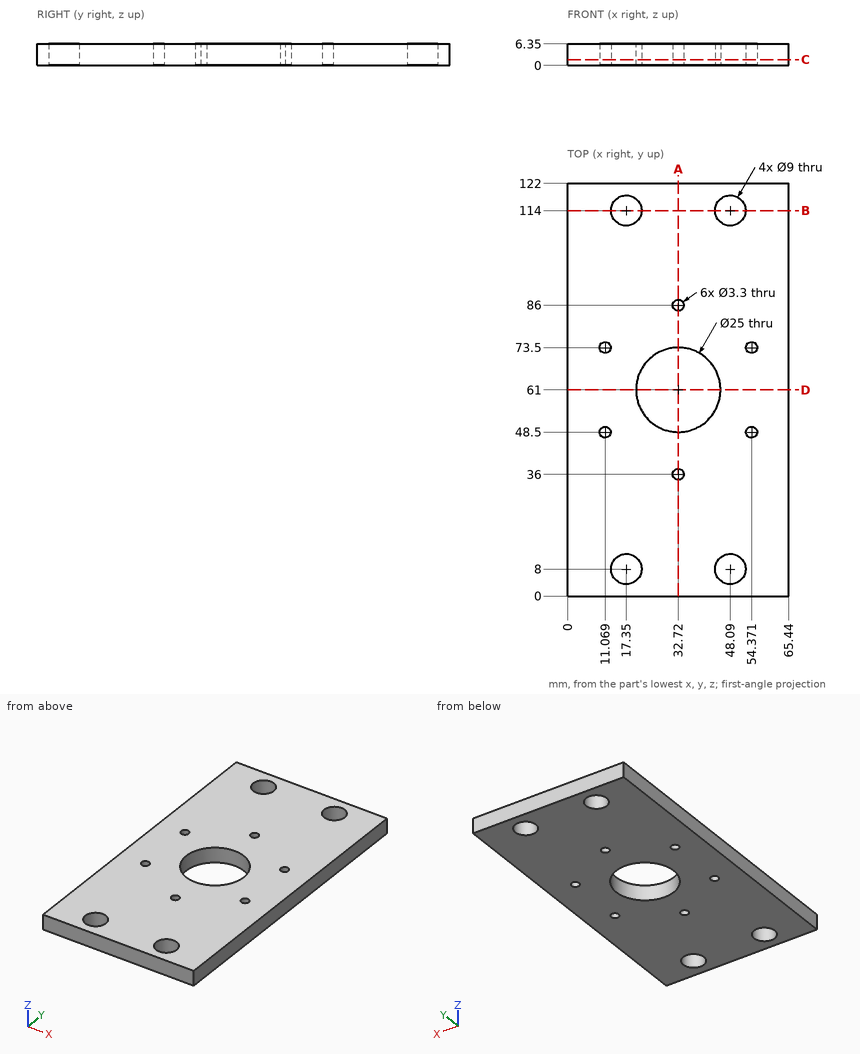
Study the drawing (mm; zero at the part's minimum x, y, z) and answer. Coordinates: 2 decimals unless noted, no trailing zeros. Write each loop counter-clockwise with the first axis right and the second up, starting at its lowest first coordinate (ties: lowest second). Pieces come first, ordered by that corner, then holes.
Q1. Section D-D, the plane y = 61 is taken. Write down the section's boundary in (x, z).
Returned:
outline: (0, 0) - (20.22, 0) - (20.22, 6.35) - (0, 6.35) - close; (45.22, 0) - (65.44, 0) - (65.44, 6.35) - (45.22, 6.35) - close
Q2. Find the intervals of material crossed by line 1 along Y through (x, z) = (17.35, 1.5); line 2 along Y through (x, z) = (32.72, 3.25); line 3 along X through (y, z) = (7.5, 1.25), in increasing order.
Returned:
line 1: y = 0 to 3.5, 12.5 to 109.5, 118.5 to 122
line 2: y = 0 to 34.35, 37.65 to 48.5, 73.5 to 84.35, 87.65 to 122
line 3: x = 0 to 12.88, 21.82 to 43.62, 52.56 to 65.44
Q3. Section B-B, the plane y = 114 is taken. Write down the section's boundary in (x, z), then the cut area to 3 significant figures.
Returned:
outline: (0, 0) - (12.85, 0) - (12.85, 6.35) - (0, 6.35) - close; (21.85, 0) - (43.59, 0) - (43.59, 6.35) - (21.85, 6.35) - close; (52.59, 0) - (65.44, 0) - (65.44, 6.35) - (52.59, 6.35) - close
area: 301 mm2
Q4. Section C-C, the plane z = 1.75 is taken. Give the number of separate pieces and of enclosed holes in the cut face, then the cut area to 3 significant figures.
Returned:
separate pieces: 1
enclosed holes: 11
area: 7,190 mm2
Q5. Section A-A, the plane x = 32.72 is taken. Write down the section's boundary in (y, z), then the cut area to 3 significant figures.
Returned:
outline: (0, 0) - (34.35, 0) - (34.35, 6.35) - (0, 6.35) - close; (37.65, 0) - (48.5, 0) - (48.5, 6.35) - (37.65, 6.35) - close; (73.5, 0) - (84.35, 0) - (84.35, 6.35) - (73.5, 6.35) - close; (87.65, 0) - (122, 0) - (122, 6.35) - (87.65, 6.35) - close
area: 574 mm2
